Here's how the part is built. I have some questions about the finished solid (model axes, mm). A direction names the side the tool comes from. Coordinates: 2 decimals unless noted, no trailing zeros. Order: outer loops, then holes, each group sorted by start corner. A loop starts at its lowest first (then second) coordinate and runs counter-clockwise, first axis right, second up. Notation, with made-up numbers: M 46.25,89 L 62.25,89 A14 cw 62.25,111 Z; hole C 63,3 d1. An arc over 180 degrees is marked long. Answer as CSV lines item,"result". Start each with the question number.
Autodesk Inventor part; units mm, degrees
ref_plane "YZ Plane" through (0, 0, 0) normal (1, 0, 0) x (0, 1, 0)
ref_plane "XZ Plane" through (0, 0, 0) normal (0, 1, 0) x (-1, 0, 0)
ref_plane "XY Plane" through (0, 0, 0) normal (0, 0, 1) x (1, 0, 0)
sketch "Sketch1" plane through (0, 0, 0) normal (0, 0, 1) x (1, 0, 0)
  line L0 (-4.7625, -2.7496) -> (-4.7625, 2.7496)
  line L1 (-4.7625, 2.7496) -> (0, 5.4993)
  line L2 (0, 5.4993) -> (4.7625, 2.7496)
  line L3 (4.7625, 2.7496) -> (4.7625, -2.7496)
  line L4 (4.7625, -2.7496) -> (0, -5.4993)
  line L5 (0, -5.4993) -> (-4.7625, -2.7496)
  point P0 (0, 0)
  point P1 (0, 0)
  dimension "Size" = 9.525
extrude "Extrusion1" add sketch "Sketch1" along normal mid plane 66.675
sketch "Sketch3" plane through (0, 0, 33.3375) normal (0, 0, 1) x (1, 0, 0)
  line L0 (-4.7625, 2.7496) -> (0, 5.4993) construction
  line L1 (0, 5.4993) -> (4.7625, 2.7496) construction
  line L2 (4.7625, 2.7496) -> (4.7625, -2.7496) construction
  line L3 (4.7625, -2.7496) -> (0, -5.4993) construction
  line L4 (0, -5.4993) -> (-4.7625, -2.7496) construction
  line L5 (-4.7625, -2.7496) -> (-4.7625, 2.7496) construction
  point P0 (0, 0)
hole "Hole1" at (0, 0, 33.3375) direction (0, 0, -1) diameter 4.4958 end through all
sketch "Sketch4" plane through (0, 0, 33.3375) normal (0, 0, 1) x (1, 0, 0)
  circle A0 centre (0, 0) radius 2.2479 construction
  line L0 (-4.7625, 2.7496) -> (0, 5.4993) construction
  line L1 (0, 5.4993) -> (4.7625, 2.7496) construction
  line L2 (4.7625, 2.7496) -> (4.7625, -2.7496) construction
  line L3 (4.7625, -2.7496) -> (0, -5.4993) construction
  line L4 (0, -5.4993) -> (-4.7625, -2.7496) construction
  line L5 (-4.7625, -2.7496) -> (-4.7625, 2.7496) construction
  circle A1 centre (0, 0) radius 5.1245
  circle A2 centre (0, 0) radius 8.89
  dimension "thunder" = 10.2489
  dimension "d16" = 17.78
extrude "Extrusion3" cut sketch "Sketch4" against normal through all
sketch "Sketch5" plane through (0, 0, 33.3375) normal (0, 0, 1) x (1, 0, 0)
  circle A0 centre (0, 0) radius 2.2479
  circle A1 centre (0, 0) radius 4.7625
  line L0 (4.7625, -1.8917) -> (4.7625, 1.8917)
  line L1 (4.0195, 3.1786) -> (0.743, 5.0703)
  line L2 (-0.743, 5.0703) -> (-4.0195, 3.1786)
  line L3 (-4.7625, 1.8917) -> (-4.7625, -1.8917)
  line L4 (-4.0195, -3.1786) -> (-0.743, -5.0703)
  line L5 (0.743, -5.0703) -> (4.0195, -3.1786)
  circle A2 centre (0, 0) radius 2.2479
  arc A3 (4.0195, -3.1786) -> (4.7625, -1.8917) centre (0, 0) ccw
  arc A4 (4.7625, 1.8917) -> (4.0195, 3.1786) centre (0, 0) ccw
  arc A5 (0.743, 5.0703) -> (-0.743, 5.0703) centre (0, 0) ccw
  arc A6 (-4.0195, 3.1786) -> (-4.7625, 1.8917) centre (0, 0) ccw
  arc A7 (-4.7625, -1.8917) -> (-4.0195, -3.1786) centre (0, 0) ccw
  arc A8 (-0.743, -5.0703) -> (0.743, -5.0703) centre (0, 0) ccw
  point P0 (2.3813, -4.1244)
  point P1 (-2.3813, -4.1244)
  point P2 (-4.7625, 0)
  point P3 (-2.3813, 4.1244)
  point P4 (2.3812, 4.1244)
  point P5 (4.7625, 0)
  dimension "d21" = 9.525
extrude "Extrusion4" cut sketch "Sketch5" against normal blind 7.9248 contours L0 A3 L5 A1 | A1 L1 A4 L0 | A1 L2 A5 L1 | L5 A8 L4 A1 | A1 L3 A6 L2 | L4 A7 L3 A1
mirror "Mirror2" about plane through (0, 0, 0) normal (0, 0, 1) of "Extrusion4"
equation "\"bearing\" = 25.4"
properties part number "GP10-008" material "Aluminum 6061"
1) Suppose I cut it at A-A on x = 0. Please give me the cut outline in (y, z).
2) Which directions (+Z, -Z, +X, -X, +Y, -Y) give clear straight access to the entire face, cutting with the end or side of a thin tool? Please do faces 1 (the face through (-4.3, -2.5, 25.413)), 2 (the face through (-3.78, 2.9, -29.43)), 3 (the face through (-4.3, 2.4, 25.413)).
3) Suppose I cut it at B-B on y = -1.25. Please give me the cut outline in (x, z), plus the area to 3 significant figures.
4) Suppose I cut it at C-C on z = -22. Please give me the cut outline in (x, y).
5) I need wall thicknesses on line 1 (X direction, y = 0, z = 0); line 2 (X direction, y = -1.25, z = -25); line 3 (Y direction, x = 1.25, z = 24). Which ranges of each line are inside material? Lowest first, please. Write a range as [from, to].
Output:
1,outline,"M -5.12,-25.41 L -4.76,-25.41 L -4.76,-33.34 L -2.25,-33.34 L -2.25,33.34 L -4.76,33.34 L -4.76,25.41 L -5.12,25.41 Z; M 2.25,-33.34 L 4.76,-33.34 L 4.76,-25.41 L 5.12,-25.41 L 5.12,25.41 L 4.76,25.41 L 4.76,33.34 L 2.25,33.34 Z"
2,face 1,"+Z, -X, -Y"
2,face 2,"-Z"
2,face 3,"+Z, -X, +Y"
3,outline,"M -4.76,-25.41 L -4.6,-25.41 L -4.6,-33.34 L -1.87,-33.34 L -1.87,33.34 L -4.6,33.34 L -4.6,25.41 L -4.76,25.41 Z; M 1.87,-33.34 L 4.6,-33.34 L 4.6,-25.41 L 4.76,-25.41 L 4.76,25.41 L 4.6,25.41 L 4.6,33.34 L 1.87,33.34 Z"
3,area,"381 mm²"
4,outline,"M -4.76,-1.89 A5.12 ccw -4.02,-3.18 L -0.74,-5.07 A5.12 ccw 0.74,-5.07 L 4.02,-3.18 A5.12 ccw 4.76,-1.89 L 4.76,1.89 A5.12 ccw 4.02,3.18 L 0.74,5.07 A5.12 ccw -0.74,5.07 L -4.02,3.18 A5.12 ccw -4.76,1.89 Z; hole C 0,0 d4.5"
5,line 1,"[-4.76, -2.25], [2.25, 4.76]"
5,line 2,"[-4.76, -1.87], [1.87, 4.76]"
5,line 3,"[-4.78, -1.87], [1.87, 4.78]"
